The listing builds one solid part. Answer for the finished solid, in the listing's coordinates (mm). Coordinates: 2 decimals unless noted, no trailing zeros. Write each loop counter-clockwise with the first axis right and the second up, starting at its lowest first coordinate (ties: lowest second). Pieces come first, ordered by that corner, then holes.
from build123d import *

# Parameters (mm, degrees)
BOSS_EXTRUDE1_DEPTH      = 152.4
BOSS_EXTRUDE1_DEPTH_BACK = 152.4
FILLET1_R                = 0.635
FILLET2_R                = 0.15875


with BuildPart() as part:
    # Sketch3 → Boss-Extrude1 (new, two sides: drawn at the far end of the back side and taken through both)
    with BuildSketch(Plane.XY.offset(-BOSS_EXTRUDE1_DEPTH_BACK)):
        Polygon((14.224, -21.8948), (14.224, 21.8948), (12.954, 21.8948), (12.954, 0.635), (-12.954, 0.635), (-12.954, 21.8948), (-14.224, 21.8948), (-14.224, -21.8948), (-12.954, -21.8948), (-12.954, -0.635), (12.954, -0.635), (12.954, -21.8948), align=None)
    extrude(amount=BOSS_EXTRUDE1_DEPTH + BOSS_EXTRUDE1_DEPTH_BACK)

    # Fillet1
    fillet1_edges = [part.edges().sort_by_distance(p)[0] for p in [
        (12.954, -0.635, 0),
        (-12.954, -0.635, 0),
        (-12.954, 0.635, 0),
        (12.954, 0.635, 0),
    ]]
    fillet(fillet1_edges, radius=FILLET1_R)

    # Fillet2
    fillet2_edges = [part.edges().sort_by_distance(p)[0] for p in [
        (12.954, -21.8948, 0),
        (-12.954, -21.8948, 0),
        (-14.224, -21.8948, 0),
        (-14.224, 21.8948, 0),
        (-12.954, 21.8948, 0),
        (12.954, 21.8948, 0),
        (14.224, 21.8948, 0),
        (14.224, -21.8948, 0),
    ]]
    fillet(fillet2_edges, radius=FILLET2_R)


solid = part.part
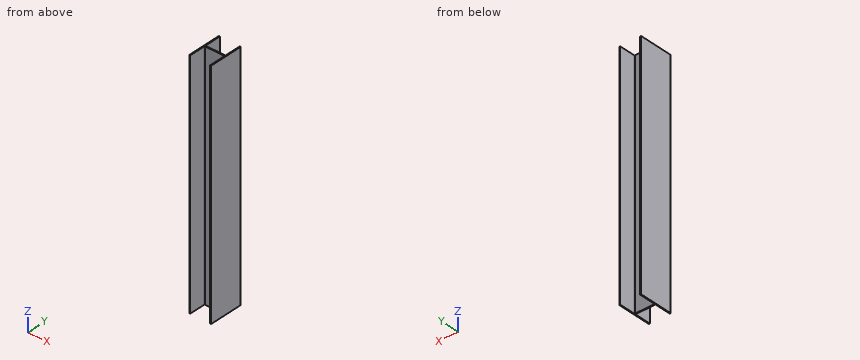
Q1. The part is cut by section C-C, the plane x = 1.5. Write down the section's boundary in (y, z) (3 decimals).
Answers below:
outline: (-0.635, -152.4) - (0.635, -152.4) - (0.635, 152.4) - (-0.635, 152.4) - close
Q2. Find the intervals of material crossed by probe 1 along X at (y, z) = (12.5, 71); probe 2 along X at (y, z) = (-1, 102.5); probe 3 along Y at (x, z) = (5.75, -125.5) (3 decimals), in increasing order.
Answers below:
probe 1: x = -14.22 to -12.95, 12.95 to 14.22
probe 2: x = -14.22 to -12.89, 12.89 to 14.22
probe 3: y = -0.635 to 0.635
Q3. Given pin 1 (10 mm diameter, centred on x = 7, z = 51, fed in from -Y) (3 decimals), flat-ended and moving along its own axis, determine where the tip first touches the part or whether it passes through.
Answers below:
pin 1: stops at y = -0.635
Q4. The part is cut by section A-A, the plane y = 11. Write down the section's boundary in (x, z), then the cut area to 3 significant figures.
Answers below:
outline: (-14.22, -152.4) - (-12.95, -152.4) - (-12.95, 152.4) - (-14.22, 152.4) - close; (12.95, -152.4) - (14.22, -152.4) - (14.22, 152.4) - (12.95, 152.4) - close
area: 774 mm2
